from build123d import *

# Parameters (mm, degrees)
SKETCH2_R                = 12.7
SOLID_CYLINDER_DEPTH     = 39.878
ALL_THROUGH_HOLE_REACH   = 45.736
SKETCH3_R                = 1.7272
SKETCH4_R                = 6.7691
SWIRL_CHAMBER_DEPTH      = 19.05
TOP_START                = -10.16
SKETCH5_R                = 12.7
SKETCH5_R_2              = 8.0391
TOP_OUTER_CUT_DEPTH      = 10.16
SKETCH8_W                = 2.286
SKETCH8_H                = 2.794
SKETCH9_W                = 4.699
SKETCH9_H                = 24.384
INNER_CHAMFER_SIZE       = 5.08
INLET_HOLE_REACH         = 45.736
INLET_HOLE_END_RADIUS    = 8.0391
SKETCH12_R               = 1.905
INLET_HOLE_PATTERN_COUNT = 4


with BuildPart() as part:
    # Sketch2 → Solid Cylinder (new body)
    with BuildSketch(Plane(origin=(0, 0, 0), x_dir=(1, 0, 0), z_dir=(0, 1, 0))):
        with Locations(Location((0, 0, 0), (0, 0, 270))):
            Circle(SKETCH2_R)
    extrude(amount=SOLID_CYLINDER_DEPTH)

    # Sketch3 → All Through Hole (cut, up to next)
    with BuildSketch(Plane(origin=(0, 39.878, 0), x_dir=(1, 0, 0), z_dir=(0, 1, 0)), mode=Mode.PRIVATE) as all_through_hole_sk1:
        with Locations(Location((0, 0, 0), (0, 0, 270))):
            Circle(SKETCH3_R)
    all_through_hole_tool1 = extrude(all_through_hole_sk1.sketch, amount=-ALL_THROUGH_HOLE_REACH, mode=Mode.PRIVATE) & part.part
    add(all_through_hole_tool1.solids().sort_by_distance((0, 39.878, 0))[0], mode=Mode.SUBTRACT)

    # Sketch4 → Swirl Chamber (cut)
    with BuildSketch(Plane(origin=(0, 39.878, 0), x_dir=(1, 0, 0), z_dir=(0, 1, 0))):
        with Locations(Location((0, 0, 0), (0, 0, 270))):
            Circle(SKETCH4_R)
    extrude(amount=-SWIRL_CHAMBER_DEPTH, mode=Mode.SUBTRACT)

    # Sketch5 → Top Outer cut (cut)
    with BuildSketch(Plane(origin=(0, 39.878, 0), x_dir=(1, 0, 0), z_dir=(0, 1, 0)).offset(TOP_START)):
        with Locations(Location((0, 0, 0), (0, 0, 270))):
            Circle(SKETCH5_R)
        with Locations(Location((0, 0, 0), (0, 0, 270))):
            Circle(SKETCH5_R_2, mode=Mode.SUBTRACT)
    extrude(amount=TOP_OUTER_CUT_DEPTH, mode=Mode.SUBTRACT)

    # Sketch8 → O Ring Cut (revolve, cut)
    with BuildSketch(Plane.XY, mode=Mode.PRIVATE) as o_ring_cut_sk:
        with Locations((11.557, 27.051)):
            Rectangle(SKETCH8_W, SKETCH8_H)
    revolve(o_ring_cut_sk.sketch.rotate(Axis((0, 55, 0), (0, -1, 0)), 90), axis=Axis((0, 55, 0), (0, -1, 0)), mode=Mode.SUBTRACT)

    # Sketch9 → Base Support (revolve, cut)
    with BuildSketch(Plane.XY, mode=Mode.PRIVATE) as base_support_sk:
        with Locations((10.3505, 12.192)):
            Rectangle(SKETCH9_W, SKETCH9_H)
    revolve(base_support_sk.sketch.rotate(Axis((0, 55, 0), (0, -1, 0)), 90), axis=Axis((0, 55, 0), (0, -1, 0)), mode=Mode.SUBTRACT)

    # Inner Chamfer
    # the kernel refuses this chamfer: 5.08 mm, written as the material it takes off along each edge
    with BuildSketch(Plane(origin=(0, 20.828, 0), x_dir=(0, 0, 1), z_dir=(-1, 0, 0))) as inner_chamfer_piece_1_section:
        Polygon((1.7272, -INNER_CHAMFER_SIZE), (1.7272 + INNER_CHAMFER_SIZE, 0), (1.7272, 0), align=None)
    inner_chamfer_piece_1 = revolve(axis=Axis((0, 20.828, 0), (0, 1, 0)), mode=Mode.PRIVATE)
    inner_chamfer_piece_1 = inner_chamfer_piece_1 & Plane(origin=(0, 18.244555095, 0), x_dir=(0, 0, 1), z_dir=(0, 1, 0)) * Cylinder(6.7691, 28, mode=Mode.PRIVATE)
    add(inner_chamfer_piece_1, mode=Mode.SUBTRACT)

    # Inlet Hole: up to this cylinder (the profile starts inside it)
    inlet_hole_end = Plane(origin=(0, 32.639, 0), z_dir=(0, 1, 0)) * Cylinder(INLET_HOLE_END_RADIUS, 108.5502, mode=Mode.PRIVATE)
    # Sketch12 → Inlet Hole (cut, up to the surface)
    with BuildSketch(Plane.XY, mode=Mode.PRIVATE) as inlet_hole_sk1:
        with Locations(Location((4.8641, 32.639, 0), (0, 0, 180))):
            Circle(SKETCH12_R)
    inlet_hole_tool1 = extrude(inlet_hole_sk1.sketch, amount=INLET_HOLE_REACH, mode=Mode.PRIVATE) & inlet_hole_end
    inlet_hole = inlet_hole_tool1.solids().sort_by_distance((4.8641, 32.639, 0))[0]
    add(inlet_hole, mode=Mode.SUBTRACT)

    # Inlet Hole Pattern: Inlet Hole ×4 about axis
    inlet_hole_pattern_axis = Axis((0, 55, 0), (0, -1, 0))
    for i in range(1, INLET_HOLE_PATTERN_COUNT):
        add(inlet_hole.rotate(inlet_hole_pattern_axis, i * 360 / INLET_HOLE_PATTERN_COUNT), mode=Mode.SUBTRACT)

    # Sketch13 → Outer Chamfer and Stem (revolve, cut)
    with BuildSketch(Plane.XY, mode=Mode.PRIVATE) as outer_chamfer_and_stem_sk:
        Polygon((-8.001, 17.272), (-3.4544, 12.7254), (-3.4544, 0), (-8.001, 0), align=None)
    revolve(outer_chamfer_and_stem_sk.sketch.rotate(Axis((0, 46.59080533, 0), (0, -1, 0)), 270), axis=Axis((0, 46.59080533, 0), (0, -1, 0)), mode=Mode.SUBTRACT)


solid = part.part
Here's how the part is built. I have some questions about the finished solid (model axes, mm). A direction names the side the tool comes from. Coordinates: 2 decimals unless noted, no trailing zeros. Order: outer loops, then holes, each group sorted by start corner. A loop starts at its lowest first (then second) coordinate and runs counter-clockwise, first axis right, second up. Notation, with made-up numbers: M -9.5,55.25 L 48.5,55.25 A14 cw 48.5,63.25 Z; hole C 53.25,31.25 d11. An arc over 180 degrees is marked long. Answer as CSV lines item,"result". Start each with the question number.
1. I want a section at A-A, the plane y = 31.5. Write out the boundary of the cut face in (x, z).
2. I need wall thicknesses on line 1 (Y direction, x = -10.5, z = -5); line 2 (X direction, y = 29.5, z = -6); line 3 (X direction, y = 11, z = 1). Which ranges of each line are inside material? Lowest first, please. Write a range as [from, to].
3. I want a section at B-B, the plane x = -9.5. Write out the boundary of the cut face in (y, z), and give its area (3 significant figures).
4. On a 3-axis mill with a long thin cutter (end or side, diameter ignored), from which of +Z, -Z, +X, -X, +Y, -Y can I reach the whole of each face in a straight line? I mean faces 1 (the cylindrical face through (7.1, 20.88, 3.69)), 2 (the cylindrical face through (6.78, 34.73, 4.32)), 3 (the cylindrical face through (-4.274, 31.759, 6.554)). Say none if no direction works.
5. For pin 1 (4.5 mm diameter, centred on x = 4.86, y = 32.64, fed in from +Z); pin 2 (2.5 mm diameter, centred on y = 32.64, z = -4.86, fed in from -X); pin 3 (12 mm diameter, centred on x = -0.5, y = 22, fed in from +Z); pin 4 (10 mm diameter, centred on x = 3.5, z = 8, fed in from -Y), each with a flat end and sliding along its axis, tell me the tip position at first contact or that it passes through.
6. We'd pull the mould along Y, two halves only. Please class faces 4 (the flat face through (-10.4, 25.654, 1.9)), 5 (the flat face through (-10.4, 28.448, 1.9)), 6 (the cylindrical face through (3.37, 6.27, -0.75)), 7 (the flat face through (2, 0, 1)): released by +Y, released by -Y, zero draft, split by the parting line, or undercut.
7. I want a section at C-C, the plane y = 23.5. Write out the boundary of the cut face in (x, z).
8. I want a section at D-D, the plane x = 8.5. Write out the boundary of the cut face in (y, z), and give its area (3 significant figures).
Recorded:
1,outline,"M -7.31,3.34 A8.04 ccw -6.39,-4.88 L -6.39,-2.23 A6.77 cw -5.89,3.34 Z; M -4.88,6.39 L -2.23,6.39 A6.77 cw 3.34,5.89 L 3.34,7.31 A8.04 ccw Z; M -3.34,-7.31 A8.04 ccw 4.88,-6.39 L 2.23,-6.39 A6.77 cw -3.34,-5.89 Z; M 5.89,-3.34 L 7.31,-3.34 A8.04 ccw 6.39,4.88 L 6.39,2.23 A6.77 cw Z"
2,line 1,"y = [24.38, 25.65], [28.45, 29.72]"
2,line 2,"x = [-11.19, -3.13], [3.13, 11.19]"
2,line 3,"x = [-3.31, -1.41], [1.41, 3.31]"
3,outline,"M 24.38,-8.43 L 25.65,-8.43 L 25.65,-4.27 L 28.45,-4.27 L 28.45,-8.43 L 29.72,-8.43 L 29.72,8.43 L 28.45,8.43 L 28.45,4.27 L 25.65,4.27 L 25.65,8.43 L 24.38,8.43 Z"
3,area,"66.7 mm2"
4,face 1,"-Y"
4,face 2,"+Y"
4,face 3,"-X"
5,pin 1,"stops at z = 7.6"
5,pin 2,"stops at x = -7.18"
5,pin 3,"stops at z = 12.7"
5,pin 4,"stops at y = 13"
6,face 4,"undercut"
6,face 5,"undercut"
6,face 6,"zero draft"
6,face 7,"released by -Y"
7,outline,"C 0,0 d16; hole C 0,0 d13.54"
8,outline,"M 24.38,-9.44 L 25.65,-9.44 L 25.65,-6.02 L 28.45,-6.02 L 28.45,-9.44 L 29.72,-9.44 L 29.72,9.44 L 28.45,9.44 L 28.45,6.02 L 25.65,6.02 L 25.65,9.44 L 24.38,9.44 Z"
8,area,"81.6 mm2"
